Part model, mm, in its own coordinate system. A direction names the side the tool comes from. Give positions to 0.01 mm unless a question says otherwise; leave off trailing zeros. Write each loop counter-clockwise with the first axis right and the second up, starting at its lowest first coordinate (ties: lowest second). Pieces come first, ordered by that corner, then holes. Notation, with made-up numbers: (31, -34.5) - (62, -34.5) arc R15 cw to (62, -8.5) - close; hole circle Ø9 at (56, 68.5). An arc over 180 degrees is marked (long way). Answer in a Markdown table with one row per item. Add a question column.
1. Band-saw the part on D-D on z = -23.5. Write the cut outline in (x, y).
2. Which spindle directions (+Z, -Z, +X, -X, +Y, -Y) get a long thin tool onto all of the face, cutting with end or side? Do faces 4 (the flat face through (14.434, 64.713, -24.853)), 5 (the flat face through (1, 0, -21)), 6 (the flat face through (29, 45, -27)), 7 (the flat face through (1, 56, -28.54)), 8 (the flat face through (5, 26, -52)). Say none if no direction does.
3. Probe line 1 along X through (y, z) = (54, -26); line 2 along X through (y, z) = (40, -24); line 3 along Z through (x, y) = (-11, 56). List the from-to ranges inside material, lowest first.
4. Band-saw the part on A-A on x = 0. Write the cut outline in (y, z), plus the area to 3 significant figures.
5. Drop flat-ended pins along their axis: pin 1 Ø0.5 at (x, z) = (-18.5, -26) entering from -Y; pin 2 Ø3.5 at (x, z) = (1, -42.5) entering from -Y; pin 3 Ø8 at (x, y) = (-14, 38) entering from -Z; pin 4 Ø6 at (x, z) = (16.5, -32.5) entering from +Y. Give the stop position or say it passes through.
6. Band-saw the part on B-B on y = 53.5. Write the cut outline in (x, z), plus the area to 3 significant figures.
7. Band-saw the part on C-C on y = 38. Write the cut outline in (x, z), plus the area to 3 significant figures.
8. Pull direction Z, two halves, no side cores. Call faces 1 (the flat face through (-26, 45, -27)), 2 (the flat face through (0.73, 66.76, -31.04)), 3 (the flat face through (4.555, 41.668, -50.306)): released by +Z, released by -Z, zero draft, split by the parting line, or undercut.
```python
from build123d import *

# Parameters (mm, degrees)
BOSS_EXTRUDE1_DEPTH     = 70
CUT_EXTRUDE1_DEPTH      = 25
CUT_EXTRUDE4_DEPTH      = 24
CUT_EXTRUDE4_DEPTH_BACK = 27
SHELL2_T                = -1
FILLET1_R               = 10
CUT_EXTRUDE3_DEPTH      = 26
CUT_EXTRUDE2_DEPTH      = 1
BOSS_EXTRUDE4_DEPTH     = 21.5
BOSS_EXTRUDE5_DEPTH     = 22
CUT_EXTRUDE8_DEPTH      = 20
CUT_EXTRUDE10_DEPTH     = 34


with BuildPart() as part:
    # Sketch2 → Boss-Extrude1 (new body)
    with BuildSketch(Plane(origin=(0, 0, 0), x_dir=(1, 0, 0), z_dir=(0, 1, 0))):
        Polygon((-18.988562983, 28.382917999), (-4.988562983, 29.470238095), (-1.988562983, 72.470238095), (4.011437017, 72.470238095), (7.011437017, 29.470238095), (32.511437017, 27.489762205), (32.511437017, 20.489762205), (-30.488562983, 20.489762205), (-30.488562983, 27.489762205), align=None)
    extrude(amount=BOSS_EXTRUDE1_DEPTH)

    # Sketch3 → Cut-Extrude1 (cut)
    with BuildSketch(Plane(origin=(0, 70, 0), x_dir=(1, 0, 0), z_dir=(0, 1, 0))):
        Polygon((-30.488562983, 27.489762205), (-30.488562983, 20.489762205), (-18.988562983, 20.489762205), (-18.988562983, 28.382917999), align=None)
        Polygon((21.011437017, 20.489762205), (32.511437017, 20.489762205), (32.511437017, 27.489762205), (21.011437017, 28.382917999), align=None)
    extrude(amount=-CUT_EXTRUDE1_DEPTH, mode=Mode.SUBTRACT)

    # Sketch7 → Cut-Extrude4 (cut, two sides: drawn at the far end of the back side and taken through both)
    with BuildSketch(Plane(origin=(0, 0, 0), x_dir=(0, 0, -1), z_dir=(1, 0, 0)).offset(-CUT_EXTRUDE4_DEPTH_BACK)):
        Polygon((20.489762205, 65), (50.489762205, 70), (20.489762205, 70), align=None)
        Polygon((72.470238095, 63), (50.489762205, 70), (72.470238095, 70), align=None)
    extrude(amount=CUT_EXTRUDE4_DEPTH + CUT_EXTRUDE4_DEPTH_BACK, mode=Mode.SUBTRACT)

    # Shell2
    shell2_openings = [part.faces().sort_by_distance(p)[0] for p in [
        (1.011437017, 0, -34.888692943),
    ]]
    offset(amount=SHELL2_T, openings=shell2_openings, kind=Kind.INTERSECTION)

    # Fillet1
    fillet1_edges = [part.edges().sort_by_distance(p)[0] for p in [
        (1.011437017, 70, -50.489762205),
    ]]
    fillet(fillet1_edges, radius=FILLET1_R)

    # Sketch6 → Cut-Extrude3 (cut)
    with BuildSketch(Plane.XZ):
        Polygon((-4.988562983, -29.470238095), (7.011437017, -29.470238095), (4.011437017, -72.470238095), (-1.988562983, -72.470238095), align=None)
    extrude(amount=-CUT_EXTRUDE3_DEPTH, mode=Mode.SUBTRACT)

    # Sketch4 → Cut-Extrude2 (cut)
    with BuildSketch(Plane(origin=(0, 45, 0), x_dir=(1, 0, 0), z_dir=(0, 1, 0))):
        Polygon((31.511437017, 21.489762205), (21.011437017, 21.489762205), (21.011437017, 27.379906551), (31.511437017, 26.564416479), align=None)
        Polygon((-29.488562983, 21.489762205), (-29.488562983, 26.564416479), (-18.988562983, 27.379906551), (-18.988562983, 21.489762205), align=None)
    extrude(amount=-CUT_EXTRUDE2_DEPTH, mode=Mode.SUBTRACT)

    # Sketch16 → Boss-Extrude4 (add)
    with BuildSketch(Plane(origin=(0, 45, 0), x_dir=(-1, 0, 0), z_dir=(0, -1, 0))):
        Polygon((-6.009006224, 29.470238095), (3.986132189, 29.470238095), (4.051029671, 28.540040848), (-6.073903706, 28.540040848), align=None)
    extrude(amount=-BOSS_EXTRUDE4_DEPTH)

    # Sketch19 → Boss-Extrude5 (add)
    with BuildSketch(Plane(origin=(0, 45, 0), x_dir=(-1, 0, 0), z_dir=(0, -1, 0))):
        Polygon((5.988562983, 28.389560926), (5.988562983, 21.489762205), (6.988562983, 21.489762205), (6.988562983, 28.311895205), align=None)
        Polygon((-8.011437017, 21.489762205), (-8.011437017, 28.389560926), (-9.011437017, 28.311895205), (-9.011437017, 21.489762205), align=None)
    extrude(amount=-BOSS_EXTRUDE5_DEPTH)

    # Sketch20 → Cut-Extrude8 (cut, symmetric)
    with BuildSketch(Plane(origin=(-5.988562983, 0, 0), x_dir=(0, 0, -1), z_dir=(1, 0, 0))):
        Polygon((21.489762205, 67), (21.489762205, 65.166666667), (30.609777223, 66.68666917), (30.609777223, 67), align=None)
    extrude(amount=CUT_EXTRUDE8_DEPTH, both=True, mode=Mode.SUBTRACT)

    # Sketch22 → Cut-Extrude10 (cut)
    with BuildSketch(Plane(origin=(0, 45, 0), x_dir=(-1, 0, 0), z_dir=(0, -1, 0))):
        Polygon((-8.011437017, 28.389560926), (-8.011437017, 20.489762205), (5.988562983, 20.489762205), (5.988562983, 28.389560926), (4.051029671, 28.540040848), (-6.073903706, 28.540040848), align=None)
    extrude(amount=-CUT_EXTRUDE10_DEPTH, mode=Mode.SUBTRACT)


solid = part.part
```
Values:
| question | item | result |
|---|---|---|
| 1 | outline | (-30.49, 0) - (-29.49, 0) - (-29.49, 45) - (-30.49, 45) - close; (-18.99, 44) - (-17.99, 44) - (-17.99, 64.49) - (-6.99, 64.49) - (-6.99, 45) - (-5.99, 45) - (-5.99, 65.5) - (-18.99, 65.5) - close; (8.01, 45) - (9.01, 45) - (9.01, 64.49) - (20.01, 64.49) - (20.01, 44) - (21.01, 44) - (21.01, 65.5) - (8.01, 65.5) - close; (31.51, 0) - (32.51, 0) - (32.51, 45) - (31.51, 45) - close |
| 2 | face 4 | -Y |
| 2 | face 5 | +Z, -Z, +X, -X, -Y |
| 2 | face 6 | +Z, -Z, +X, +Y |
| 2 | face 7 | +Z, +Y, -Y |
| 2 | face 8 | -Z, +X, -X, -Y |
| 3 | line 1 | x = -18.99 to -17.99, -6.99 to -5.99, 8.01 to 9.01, 20.01 to 21.01 |
| 3 | line 2 | x = -30.49 to -29.49, 31.51 to 32.51 |
| 3 | line 3 | z = -29 to -28, -21.49 to -20.49 |
| 4 | outline | (0, -21.49) - (45, -21.49) - (45, -20.49) - (0, -20.49) - close; (26, -72.47) - (63, -72.47) - (69.27, -52.79) arc R10 ccw to (69.6, -48.11) - (66.34, -28.54) - (45, -28.54) - (45, -29.47) - (65.48, -29.47) - (68.97, -50.42) - (62.27, -71.47) - (26, -71.47) - close |
| 4 | area | 145 mm² |
| 5 | pin 1 | stops at y = 44 |
| 5 | pin 2 | stops at y = 67.36 |
| 5 | pin 3 | stops at z = -29.08 |
| 5 | pin 4 | passes through |
| 6 | outline | (-18.99, -28.38) - (-4.99, -29.47) - (-1.99, -72.47) - (4.01, -72.47) - (7.01, -29.47) - (21.01, -28.38) - (21.01, -20.49) - (8.01, -20.49) - (8.01, -28.39) - (6.07, -28.54) - (-4.05, -28.54) - (-5.99, -28.39) - (-5.99, -20.49) - (-18.99, -20.49) - close; hole (-17.99, -27.46) - (-6.99, -28.31) - (-6.99, -21.49) - (-17.99, -21.49) - close; hole (-3.99, -29.47) - (-1.06, -71.47) - (3.08, -71.47) - (6.01, -29.47) - close; hole (9.01, -28.31) - (20.01, -27.46) - (20.01, -21.49) - (9.01, -21.49) - close |
| 6 | area | 181 mm² |
| 7 | outline | (-30.49, -27.49) - (-4.99, -29.47) - (-1.99, -72.47) - (4.01, -72.47) - (7.01, -29.47) - (32.51, -27.49) - (32.51, -20.49) - (-30.49, -20.49) - close; hole (-29.49, -26.56) - (-4.05, -28.54) - (-1.06, -71.47) - (3.08, -71.47) - (6.07, -28.54) - (31.51, -26.56) - (31.51, -21.49) - (-29.49, -21.49) - close |
| 7 | area | 216 mm² |
| 8 | face 1 | zero draft |
| 8 | face 2 | released by +Z |
| 8 | face 3 | undercut |
